from build123d import *

# Parameters (mm, degrees)
BOSS_EXTRUDE1_DEPTH = 5
CUT_EXTRUDE1_DEPTH  = 20
CUT_EXTRUDE2_DEPTH  = 20
CUT_EXTRUDE3_DEPTH  = 15.5
CUT_EXTRUDE4_DEPTH  = 15.5
SKETCH6_W           = 15
SKETCH6_H           = 32.5
CUT_EXTRUDE5_DEPTH  = 3
FILLET1_R           = 3
SKETCH7_W           = 15
SKETCH7_H           = 2.5
BOSS_EXTRUDE2_DEPTH = 2
FILLET2_R           = 3
FILLET3_R           = 3
CUT_EXTRUDE6_DEPTH  = 5
BOSS_EXTRUDE3_DEPTH = 5
CUT_EXTRUDE7_DEPTH  = 5
CUT_EXTRUDE8_DEPTH  = 5
FILLET4_R           = 2
FILLET5_R           = 2


# Some blends are built 0.0001 mm under size
with BuildPart() as part:
    # Sketch1 → Boss-Extrude1 (new body)
    with BuildSketch(Plane.XY):
        Polygon((0, 0), (0, 144.5), (20, 144.5), (20, 150), (35.5, 150), (35.5, 115), (36.5, 115), (36.5, 150), (51.5, 150), (51.5, 115), (52.5, 115), (52.5, 150), (68, 150), (68, 144.5), (88, 144.5), (88, 0), align=None)
    extrude(amount=BOSS_EXTRUDE1_DEPTH)

    # Sketch2 → Cut-Extrude1 (cut)
    with BuildSketch(Plane(origin=(88, 0, 0), x_dir=(0, 0, -1), z_dir=(1, 0, 0))):
        Polygon((-5, 144.5), (0, 144.5), (-5, 143.253359986), align=None)
    extrude(amount=-CUT_EXTRUDE1_DEPTH, mode=Mode.SUBTRACT)

    # Sketch3 → Cut-Extrude2 (cut)
    with BuildSketch(Plane.ZY):
        Polygon((5, 144.5), (0, 144.5), (5, 143.253359986), align=None)
    extrude(amount=-CUT_EXTRUDE2_DEPTH, mode=Mode.SUBTRACT)

    # Sketch4 → Cut-Extrude3 (cut)
    with BuildSketch(Plane(origin=(68, 0, 0), x_dir=(0, 0, -1), z_dir=(1, 0, 0))):
        Polygon((0, 150), (-5, 148.753359986), (-5, 150), align=None)
    extrude(amount=-CUT_EXTRUDE3_DEPTH, mode=Mode.SUBTRACT)

    # Sketch5 → Cut-Extrude4 (cut)
    with BuildSketch(Plane.ZY.offset(-20)):
        Polygon((0, 150), (5, 150), (5, 148.753359986), align=None)
    extrude(amount=-CUT_EXTRUDE4_DEPTH, mode=Mode.SUBTRACT)

    # Sketch6 → Cut-Extrude5 (cut)
    with BuildSketch(Plane.XY.offset(5)):
        with Locations((44, 131.25)):
            Rectangle(SKETCH6_W, SKETCH6_H)
    extrude(amount=-CUT_EXTRUDE5_DEPTH, mode=Mode.SUBTRACT)

    # Fillet1
    fillet1_edges = [part.edges().sort_by_distance(p)[0] for p in [
        (44, 115, 2),
    ]]
    fillet(fillet1_edges, radius=FILLET1_R - 0.0001)  # a hair under: the kernel refuses the full size

    # Sketch7 → Boss-Extrude2 (add)
    with BuildSketch(Plane.XY.offset(5)):
        with Locations((44, 148.75)):
            Rectangle(SKETCH7_W, SKETCH7_H)
    extrude(amount=BOSS_EXTRUDE2_DEPTH)

    # Fillet2
    fillet2_edges = [part.edges().sort_by_distance(p)[0] for p in [
        (44, 147.5, 2),
    ]]
    fillet(fillet2_edges, radius=FILLET2_R)

    # Fillet3
    # the kernel refuses this fillet: 3 mm, written as the material it takes off along each edge
    with BuildSketch(Plane(origin=(58.895099729, 150, 7), x_dir=(0, -1, 0), z_dir=(-1, 0, 0))) as fillet3_piece_1:
        with BuildLine():
            CenterArc((3, -2.958039892), FILLET3_R, 99.594068227, 80.405931773)
            Line((0, -2.958039892), (-0.06, -2.958039892))
            Line((-0.06, -2.958039892), (-0.06, 0))
            Line((-0.06, 0), (0, 0.06))
            ThreePointArc((0, 0.06), (1.25, 0.06), (2.49, 0.059160798))
            Line((2.49, 0.059160798), (2.5, 0))
        make_face()
    extrude(amount=29.790199458, mode=Mode.SUBTRACT)

    # Sketch8 → Cut-Extrude6 (cut)
    with BuildSketch(Plane.XY.offset(5)):
        with BuildLine():
            Line((35, 80), (35, 35))
            ThreePointArc((35, 35), (44, 26), (53, 35))
            Line((53, 35), (53, 80))
            ThreePointArc((53, 80), (44, 89), (35, 80))
        make_face()
    extrude(amount=-CUT_EXTRUDE6_DEPTH, mode=Mode.SUBTRACT)

    # Sketch9 → Boss-Extrude3 (add)
    with BuildSketch(Plane.XY.offset(5)):
        with BuildLine():
            Line((25, 143.253359986), (25, 35.253359986))
            ThreePointArc((25, 35.253359986), (44, 16.253359986), (63, 35.253359986))
            Line((63, 35.253359986), (63, 143.253359986))
            Line((63, 143.253359986), (58, 143.253359986))
            Line((58, 143.253359986), (58, 35.253359986))
            ThreePointArc((58, 35.253359986), (44, 21.253359986), (30, 35.253359986))
            Line((30, 35.253359986), (30, 143.253359986))
            Line((30, 143.253359986), (25, 143.253359986))
        make_face()
    extrude(amount=BOSS_EXTRUDE3_DEPTH)

    # Sketch10 → Cut-Extrude7 (cut)
    with BuildSketch(Plane.ZY.offset(-25)):
        Polygon((5, 143.253359986), (10, 142.006719972), (10, 143.253359986), align=None)
    extrude(amount=-CUT_EXTRUDE7_DEPTH, mode=Mode.SUBTRACT)

    # Sketch11 → Cut-Extrude8 (cut)
    with BuildSketch(Plane(origin=(63, 0, 0), x_dir=(0, 0, -1), z_dir=(1, 0, 0))):
        Polygon((-5, 143.253359986), (-10, 142.006719972), (-10, 143.253359986), align=None)
    extrude(amount=-CUT_EXTRUDE8_DEPTH, mode=Mode.SUBTRACT)

    # Fillet4
    fillet4_edges = [part.edges().sort_by_distance(p)[0] for p in [
        (44, 16.253359986, 10),
        (63, 88.630039979, 10),
        (25, 88.630039979, 10),
    ]]
    fillet(fillet4_edges, radius=FILLET4_R)

    # Fillet5
    fillet5_edges = [part.edges().sort_by_distance(p)[0] for p in [
        (44, 21.253359986, 10),
        (30, 88.630039979, 10),
        (58, 88.630039979, 10),
    ]]
    fillet(fillet5_edges, radius=FILLET5_R)


solid = part.part
Part model, mm, in its own coordinate system. A direction names the side the tool comes from. Round coordinates to 2 decimals unless told otherwise and drop trailing zeros. Order: outer loops, then holes, each group sorted by start corner. A loop starts at its lowest first (then second) coordinate and runs counter-clockwise, first axis right, second up. Notation, with made-up numbers: (48.25, 55) -> (82.25, 55) arc R17 ccw to (82.25, 66) -> close; hole circle Ø5 at (-17, 80.25). An arc over 180 degrees is marked (long way). Put each result on its own line as item: value.
Q1. Band-saw the part on B-B (y = 83). Give the cut face in (x, z).
From the geometry:
outline: (0, 0) -> (35.51, 0) -> (35.51, 5) -> (30, 5) -> (30, 8) arc R2 ccw to (28, 10) -> (27, 10) arc R2 ccw to (25, 8) -> (25, 5) -> (0, 5) -> close; (52.49, 0) -> (88, 0) -> (88, 5) -> (63, 5) -> (63, 8) arc R2 ccw to (61, 10) -> (60, 10) arc R2 ccw to (58, 8) -> (58, 5) -> (52.49, 5) -> close
Q2. Pin check, flat tips, straight feed: pin 1 Ø0.9 at (y, z) = (111, 7) entering from +X; pin 2 Ø5.5 at (y, z) = (47.5, 1.5) entering from -X; pin 3 Ø1.5 at (y, z) = (145.5, 2) entering from -X; pin 4 Ø16.5 at (x, y) = (42, 130.5) entering from +Z. Stop position of each tip, or through.
From the geometry:
pin 1: stops at x = 63
pin 2: stops at x = 0
pin 3: stops at x = 20
pin 4: stops at z = 5
Q3. Tool access for faces 1 (the face through (20, 147, 2)), 2 (the face through (52.5, 132, 2)), 3 (the face through (30, 88, 6)), 4 (the face through (44.308, 21.257, 6.479)): list every direction of +Z, -Z, +X, -X, +Y, -Y with a clear straight run to the whole face (end or side of a thin tool).
From the geometry:
face 1: +Z, -X, +Y
face 2: +Z, -Z, +Y
face 3: +Z, +Y
face 4: +Z
Q4. Band-saw the part on C-C (x = 80). Give the cut face in (y, z), and give its area (3 significant figures).
From the geometry:
outline: (0, 0) -> (144.5, 0) -> (143.25, 5) -> (0, 5) -> close
area: 719 mm2
Q5. Wall check: line 1 (X direction, y = 116, z = 6.75); line 2 (X direction, y = 55, z = 0.75); line 3 (Y direction, x = 41.5, z = 4.75). Give the ranges that are in metal, low to high. Write a range as [from, to].
From the geometry:
line 1: x = [25, 30], [58, 63]
line 2: x = [0, 35], [53, 88]
line 3: y = [0, 26.35], [88.65, 115.01], [147.49, 149.92]
